from build123d import *

# Parameters (mm, degrees)
SCHIZZO1_R                   = 2.05
ESTRUSIONE_ESTRUSIONE1_DEPTH = 5
SCHIZZO2_R                   = 2.05
TAGLIO_ESTRUSIONE1_DEPTH     = 10
CUT_EXTRUDE1_REACH           = 7
SKETCH1_W                    = 17
SKETCH1_H                    = 5
CUT_EXTRUDE2_REACH           = 7
SKETCH2_R                    = 2.05


with BuildPart() as part:
    # Schizzo1 → Estrusione-Estrusione1 (new body)
    with BuildSketch(Plane.XY):
        with BuildLine():
            ThreePointArc((-1.538071066, 7.340595166), (-7.378454008, -1.344773756), (1.150548918, -7.411223731))
            ThreePointArc((1.150548918, -7.411223731), (75.443261143, -2.885528453), (149.288277512, -12.20231786))
            ThreePointArc((149.288277512, -12.20231786), (152.810661847, -12.473685396), (156.268292683, -11.748688334))
            ThreePointArc((156.268292683, -11.748688334), (178.283063002, -6.762377854), (200.846153846, -7.410711103))
            ThreePointArc((200.846153846, -7.410711103), (209.378154672, -1.346415107), (203.538071066, 7.340595166))
            ThreePointArc((203.538071066, 7.340595166), (101, 17.967584078), (-1.538071066, 7.340595166))
        make_face()
        Circle(SCHIZZO1_R, mode=Mode.SUBTRACT)
        with Locations((202, 0)):
            Circle(SCHIZZO1_R, mode=Mode.SUBTRACT)
        with Locations((152, 0)):
            Circle(SCHIZZO1_R, mode=Mode.SUBTRACT)
    extrude(amount=ESTRUSIONE_ESTRUSIONE1_DEPTH)

    # Schizzo2 → Taglio-Estrusione1 (cut)
    with BuildSketch(Plane.XY.offset(5)):
        with Locations((21.792647349, 3.923925867)):
            Circle(SCHIZZO2_R)
        with Locations((115.643522851, 5.673925867)):
            Circle(SCHIZZO2_R)
    extrude(amount=-TAGLIO_ESTRUSIONE1_DEPTH, mode=Mode.SUBTRACT)

    # Sketch1 → Cut-Extrude1 (cut, up to next)
    with BuildSketch(Plane.XY.offset(5), mode=Mode.PRIVATE) as cut_extrude1_sk1:
        with Locations((184, 2.320601078)):
            Rectangle(SKETCH1_W, SKETCH1_H)
    cut_extrude1_tool1 = extrude(cut_extrude1_sk1.sketch, amount=-CUT_EXTRUDE1_REACH, mode=Mode.PRIVATE) & part.part
    add(cut_extrude1_tool1.solids().sort_by_distance((184, 2.320601, 5))[0], mode=Mode.SUBTRACT)

    # Sketch2 → Cut-Extrude2 (cut, up to next)
    with BuildSketch(Plane.XY.offset(5), mode=Mode.PRIVATE) as cut_extrude2_sk1:
        with Locations((175.5, 4.820601078)):
            Circle(SKETCH2_R)
    cut_extrude2_tool1 = extrude(cut_extrude2_sk1.sketch, amount=-CUT_EXTRUDE2_REACH, mode=Mode.PRIVATE) & part.part
    add(cut_extrude2_tool1.solids().sort_by_distance((175.5, 4.820601, 5))[0], mode=Mode.SUBTRACT)
    # Sketch2 → Cut-Extrude2 (cut, up to next)
    with BuildSketch(Plane.XY.offset(5), mode=Mode.PRIVATE) as cut_extrude2_sk2:
        with Locations((175.5, -0.179398922)):
            Circle(SKETCH2_R)
    cut_extrude2_tool2 = extrude(cut_extrude2_sk2.sketch, amount=-CUT_EXTRUDE2_REACH, mode=Mode.PRIVATE) & part.part
    add(cut_extrude2_tool2.solids().sort_by_distance((175.5, -0.179399, 5))[0], mode=Mode.SUBTRACT)
    # Sketch2 → Cut-Extrude2 (cut, up to next)
    with BuildSketch(Plane.XY.offset(5), mode=Mode.PRIVATE) as cut_extrude2_sk3:
        with Locations((192.5, -0.179398922)):
            Circle(SKETCH2_R)
    cut_extrude2_tool3 = extrude(cut_extrude2_sk3.sketch, amount=-CUT_EXTRUDE2_REACH, mode=Mode.PRIVATE) & part.part
    add(cut_extrude2_tool3.solids().sort_by_distance((192.5, -0.179399, 5))[0], mode=Mode.SUBTRACT)
    # Sketch2 → Cut-Extrude2 (cut, up to next)
    with BuildSketch(Plane.XY.offset(5), mode=Mode.PRIVATE) as cut_extrude2_sk4:
        with Locations((192.5, 4.820601078)):
            Circle(SKETCH2_R)
    cut_extrude2_tool4 = extrude(cut_extrude2_sk4.sketch, amount=-CUT_EXTRUDE2_REACH, mode=Mode.PRIVATE) & part.part
    add(cut_extrude2_tool4.solids().sort_by_distance((192.5, 4.820601, 5))[0], mode=Mode.SUBTRACT)


solid = part.part
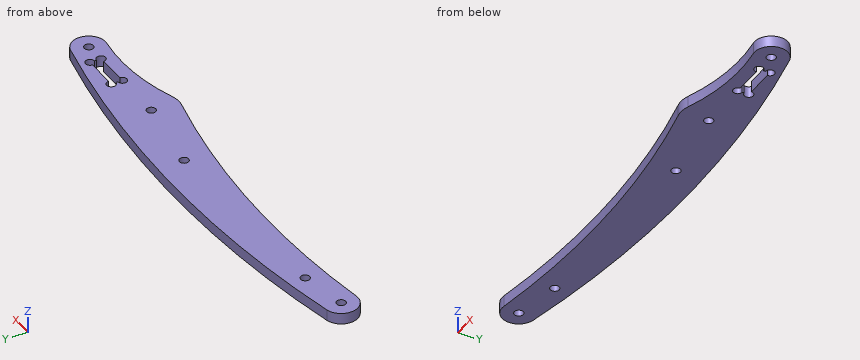
Part model, mm, in its own coordinate system. Give positions to 0.01 mm unless a question says otherwise; leave off trailing zeros. Loops run counter-clockwise (first coordinate to the right, second up) from the corner with the lowest first, then second, coordinate; pieces in that order, holes last. Notation, with made-up numbers: M 53,-37.75 L 92,-37.75 A22 ccw 92,-9.75 Z; hole C 78.5,57.25 d10. An arc over 180 degrees is marked long. Put each result on its own line as item: value. Start each with the question number.
1) Flat gauge pin, fed straight in: pin 1 (3.5 mm diameter, centred on x = 175.5, y = -0.18, fed in from +Z). Where does the tip first touch, or does it go through?
2) Probe probe 1 along X at (y, z) = (4.5, 0.85); probe 2 along Y at (x, z) = (152, 1.35); probe 3 along Y at (x, z) = (0, 3.4). List the from-to ranges inside material, lowest first.
3) Saw through at C-C (z = 0.9). List the corners of the cut face in (x, y).
4) Saw through at A-A (x = 152). List the corners of the cut face in (y, z), then the cut area to 3 significant figures.
5) Saw through at B-B (y = -4.5). List the corners of the cut face in (x, z).
Numbers:
1. pin 1: through
2. probe 1: -6 to 19.83, 23.76 to 113.96, 117.32 to 173.48, 194.52 to 208
2. probe 2: -12.5 to -2.05, 2.05 to 15.36
2. probe 3: -7.5 to -2.05, 2.05 to 7.66
3. outline: M -1.54,7.34 A7.5 ccw 1.15,-7.41 A400 cw 149.29,-12.2 A12.5 ccw 156.27,-11.75 A90 cw 200.85,-7.41 A7.5 ccw 203.54,7.34 A500 ccw Z; hole C 0,0 d4.1; hole C 21.79,3.92 d4.1; hole C 115.64,5.67 d4.1; hole C 152,0 d4.1; hole M 175.5,1.87 A2.05 ccw long 177.55,-0.18 L 190.45,-0.18 A2.05 ccw long 192.5,1.87 L 192.5,2.77 A2.05 ccw long 190.45,4.82 L 177.55,4.82 A2.05 ccw long 175.5,2.77 Z; hole C 202,0 d4.1
4. outline: M -12.5,0 L -2.05,0 L -2.05,5 L -12.5,5 Z; M 2.05,0 L 15.36,0 L 15.36,5 L 2.05,5 Z
4. area: 119 mm^2
5. outline: M -6,0 L 24.36,0 L 24.36,5 L -6,5 Z; M 100.66,0 L 208,0 L 208,5 L 100.66,5 Z
